The listing builds one solid part. Answer for the finished solid, in the listing's coordinates (mm). A direction names the side the tool comes from. Coordinates: 2 decimals unless noted, no trailing zeros. Order: outer loops, then holes, each group sorted by start corner. A loop starts at its lowest first (then second) coordinate and runs counter-clockwise, first axis right, second up.
```python
from build123d import *

# Parameters (mm, degrees)
REDONDEO1_R             = 1
REDONDEO2_R             = 1
CHAFL_N1_SIZE           = 0.3
CHAFL_N2_SIZE           = 0.5
CROQUIS2_W              = 2.564908208
CROQUIS2_H              = 0.459088629
CROQUIS2_W_2            = 0.638732005
CROQUIS2_H_2            = 2.39524502
CROQUIS2_W_3            = 0.538930129
CROQUIS2_H_3            = 2.714611022
SALIENTE_EXTRUIR1_DEPTH = 8


with BuildPart() as part:
    # Croquis1 → Revolución1 (revolve)
    with BuildSketch(Plane.XY, mode=Mode.PRIVATE) as revoluci_n1_sk:
        Polygon((0, 0), (1, 0), (1, 6), (2.75, 6), (2.75, -2.5), (3.875, -2.5), (3.875, 3), (5.425, 3), (5.425, 6), (4.25, 6), (4.25, 13), (0, 13), align=None)
    revolve(revoluci_n1_sk.sketch.rotate(Axis((0, 0, 0), (0, -1, 0)), 90), axis=Axis((0, 0, 0), (0, -1, 0)))

    # Redondeo1
    redondeo1_edges = [part.edges().sort_by_distance(p)[0] for p in [
        (0, 0, -1),
    ]]
    fillet(redondeo1_edges, radius=REDONDEO1_R)

    # Redondeo2
    redondeo2_edges = [part.edges().sort_by_distance(p)[0] for p in [
        (0, 6, -5.425),
    ]]
    fillet(redondeo2_edges, radius=REDONDEO2_R)

    # Chaflán1
    chafl_n1_edges = [part.edges().sort_by_distance(p)[0] for p in [
        (0, 3, -5.425),
        (0, -2.5, -3.875),
        (0, -2.5, -2.75),
    ]]
    chamfer(chafl_n1_edges, length=CHAFL_N1_SIZE)

    # Chaflán2
    chafl_n2_edges = [part.edges().sort_by_distance(p)[0] for p in [
        (0, 13, -4.25),
    ]]
    chamfer(chafl_n2_edges, length=CHAFL_N2_SIZE)

    # Croquis2 → Saliente-Extruir1 (add)
    with BuildSketch(Plane(origin=(0, 13, 0), x_dir=(1, 0, 0), z_dir=(0, 1, 0))):
        with Locations((0, -3.023996838)):
            Rectangle(CROQUIS2_W, CROQUIS2_H)
        with Locations((3.009026556, 0)):
            Rectangle(CROQUIS2_W_2, CROQUIS2_H_2)
        with Locations((-2.779482242, 0)):
            Rectangle(CROQUIS2_W_3, CROQUIS2_H_3)
    extrude(amount=SALIENTE_EXTRUIR1_DEPTH)


solid = part.part
```
(1) The mould has two halves that part along X. Classify faces 1 (the face through (1, 4, 0)), 2 (the face through (-4, 3, -1)), 3 (the face through (-3.049, 17, 0)): released by +X, released by -X, zero draft, split by the parting line, or undercut.
(2) Each of these flat-tipped pins is pushed along its axis until it touches: pin 1 Ø3.5 at (x, z) = (0, 0) entering from +Y; pin 2 Ø4 at (x, y) = (-3.5, 11) entering from -Z; pin 3 Ø2 at (x, y) = (-3.5, 5.5) entering from +Z. Where does it stop, or does it pass through?
(3) Consider line 1 (X direction, y = 1.25, z = 0) (3 decimals); line 2 (X direction, y = 0.5, z = 0) (3 decimals); line 3 (Y direction, x = -0.75, z = -1.5). Determine where each line is inside the solid, lowest interval first.
(4) For faces 4 (the face through (2.685, 1.843, -0.596)), 5 (the face through (3.328, 17, 0)), 6 (the face through (2.69, 17, 0)), 7 (the face through (-4.214, 9.296, -0.553)), 8 (the face through (0, 17, 2.794)), determine the directions among +Z, -Z, +X, -X, +Y, -Y from which every point of the face is accessible in a straight line to the end or side of a thin tool.
(5) Find section C-C (y = 11). Write down the section's boundary in (x, z), and give its area (3 significant figures).
(6) Find section A-A (y = 19.75). Write down the section's boundary in (x, z), and give its area (3 significant figures).
Findings below:
1. face 1: undercut
1. face 2: zero draft
1. face 3: released by -X
2. pin 1: stops at y = 13
2. pin 2: stops at z = -3.98
2. pin 3: stops at z = 4.77
3. line 1: x = -3.875 to -2.75, -1 to 1, 2.75 to 3.875
3. line 2: x = -3.875 to -2.75, -0.866 to 0.866, 2.75 to 3.875
3. line 3: y = 6 to 13
4. face 4: -Y
4. face 5: +Z, -Z, +X, +Y
4. face 6: +Z, -Z, +Y
4. face 7: +Y
4. face 8: -Z, +X, -X, +Y
5. outline: circle Ø8.5 at (0, 0)
5. area: 56.7 mm2
6. outline: (-3.05, -1.36) - (-2.51, -1.36) - (-2.51, 1.36) - (-3.05, 1.36) - close; (-1.28, 2.79) - (1.28, 2.79) - (1.28, 3.25) - (-1.28, 3.25) - close; (2.69, -1.2) - (3.33, -1.2) - (3.33, 1.2) - (2.69, 1.2) - close
6. area: 4.17 mm2
